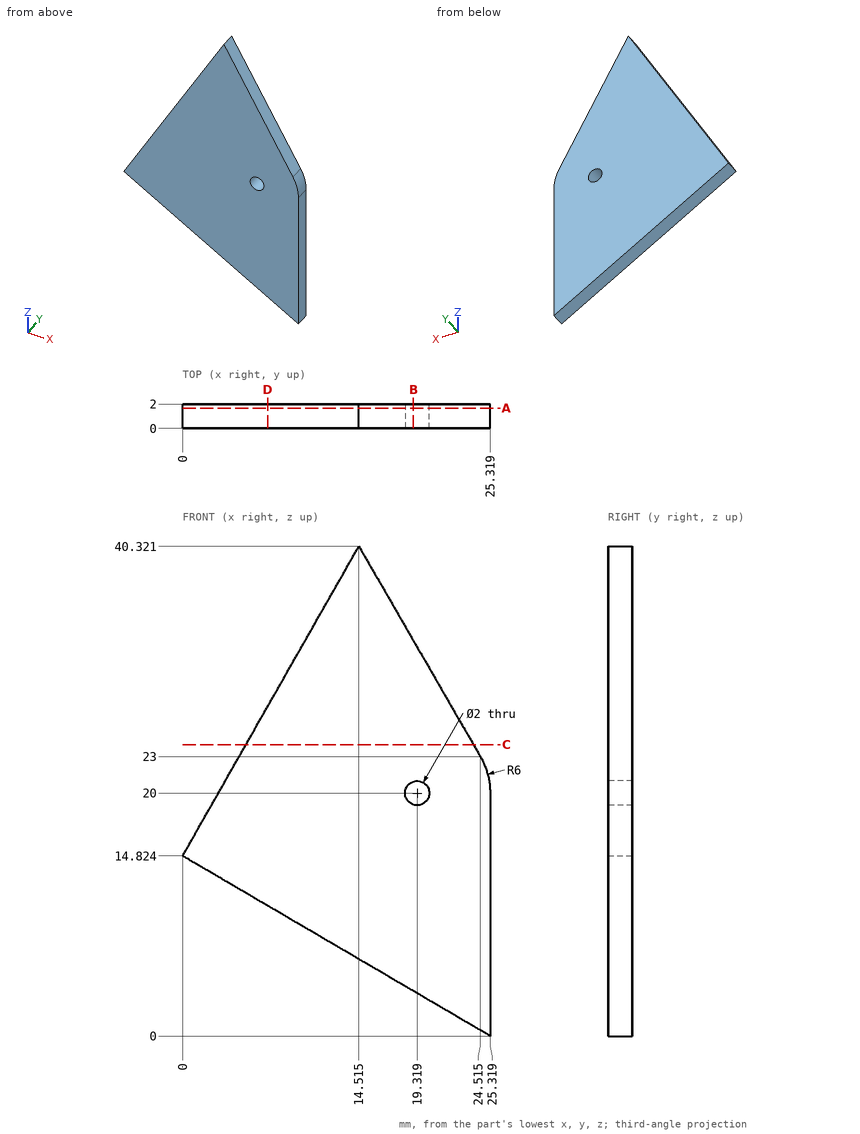
The drawing under review shows one solid part. Ordinate dimensions are in mm from its lowest x, y, z. Coordinates: 2 decimals unless noted, no trailing zeros. Loops run counter-clockwise (first coordinate to the right, second up) from the corner with the lowest first, then second, coordinate; pieces in that order, holes last.
Item 1: Add section C-C (z = 24). Write out the cut boundary in (x, y).
Completed:
outline: (5.22, 0) - (23.94, 0) - (23.94, 2) - (5.22, 2) - close
Item 2: Add section B-B (x = 19). Write out the cut boundary in (y, z).
Completed:
outline: (0, 3.7) - (2, 3.7) - (2, 19.05) - (0, 19.05) - close; (0, 20.95) - (2, 20.95) - (2, 32.55) - (0, 32.55) - close
Item 3: Add section D-D (x = 7). Write out the cut boundary in (y, z) (1 decimal).
Completed:
outline: (0, 10.7) - (2, 10.7) - (2, 27.1) - (0, 27.1) - close
Item 4: Clearance check with a flat-ended pin moving along its axis: pin 1 (1 mm diameter, centred on x = 4.5, y = 0.5, fed in from -Z) (1 decimal). State where the tip first meets the part, or that it passes through.
Completed:
pin 1: stops at z = 11.9
Item 5: Wall thickness on L1, parallel to X at y = 0.7, z = 20 (1 decimal); L2, parallel to Z at x = 10, y = 0.15 (1 decimal); L3, parallel to X at y = 1.8, z = 31.5 (1 decimal): over which ranges is each line inside the solid? List them lowest first.
Completed:
L1: x = 2.9 to 18.3, 20.3 to 25.3
L2: z = 9 to 32.4
L3: x = 9.5 to 19.6
Item 6: Add section A-A (y = 1.65). Write out the cut boundary in (x, z) (1 decimal), and give its area (3 significant figures).
Completed:
outline: (0, 14.8) - (25.3, 0) - (25.3, 20) arc R6 ccw to (24.5, 23) - (14.5, 40.3) - close; hole circle Ø2 at (19.3, 20)
area: 544 mm2
